```python
from build123d import *

# Parameters (mm, degrees)
SKETCH1_W            = 400
SKETCH1_H            = 800
BASE_DEPTH           = 18
SKETCH2_R            = 3.15
MOUNTING_HOLES_DEPTH = 19
TAP_HOLE_REACH       = 20
SKETCH4_R            = 8


with BuildPart() as part:
    # Sketch1 → Base (new body)
    with BuildSketch(Plane.XY):
        with Locations((200, 400)):
            Rectangle(SKETCH1_W, SKETCH1_H)
    extrude(amount=BASE_DEPTH)

    # Sketch2 → Mounting holes (cut, through all)
    with BuildSketch(Plane.XY.offset(18)):
        with Locations((25, 775)):
            Circle(SKETCH2_R)
        with Locations((375, 775)):
            Circle(SKETCH2_R)
        with Locations((25, 150)):
            Circle(SKETCH2_R)
        with Locations((375, 150)):
            Circle(SKETCH2_R)
    extrude(amount=-MOUNTING_HOLES_DEPTH, mode=Mode.SUBTRACT)

    # Sketch4 → Tap hole (cut, up to next)
    with BuildSketch(Plane(origin=(0, 0, 0), x_dir=(-1, 0, 0), z_dir=(0, 0, -1)), mode=Mode.PRIVATE) as tap_hole_sk1:
        with Locations((-75, 75)):
            Circle(SKETCH4_R)
    tap_hole_tool1 = extrude(tap_hole_sk1.sketch, amount=-TAP_HOLE_REACH, mode=Mode.PRIVATE) & part.part
    add(tap_hole_tool1.solids().sort_by_distance((75, 75, 0))[0], mode=Mode.SUBTRACT)


solid = part.part
```
Part model, mm, in its own coordinate system. Round coordinates to 2 decimals unless told otherwise and drop trailing zeros. Order: outer loops, then holes, each group sorted by start corner. A loop starts at its lowest first (then second) coordinate and runs counter-clockwise, first axis right, second up. Notation, with made-up numbers: M 31,-18.5 L 52,-18.5 A27 ccw 52,8.5 Z; hole C -13,41 d6. An arc over 180 degrees is marked long. Answer in a Markdown table with one row per item. Add a question column.
Q1. Cut at B-B on x = 75. Give the cut face in (y, z).
Q2. Cut at A-A on y = 75. Give the cut face in (x, z).
Q3. Pin check, flat tips, straight feed: pin 1 (5 mm diameter, centred on x = 25, y = 150, fed in from +Z); pin 2 (10 mm diameter, centred on x = 281, y = 330.5, fed in from -Z). Stop position of each tip, or through.
Q4. Wall check: L1, parallel to Y at x = 25, z = 6.25; L2, parallel to X at y = 150, z = 3.75; L3, parallel to Y at x = 69, z = 15.5. Give the ranges that are in metal, low to high. Write a range as from..to.
Q5. Mould opens along Y. For faces 1 (the face through (197, 800, 9)), 2 (the face through (197, 0, 9)), 3 (the face through (76.041, 82.932, 8.874)), 4 (the face through (197, 406, 18)) say: +Y half, -Y half, draft (parallel to the pull), parting line (faces both ways), or undercut.
Established:
| question | item | result |
|---|---|---|
| 1 | outline | M 0,0 L 67,0 L 67,18 L 0,18 Z; M 83,0 L 800,0 L 800,18 L 83,18 Z |
| 2 | outline | M 0,0 L 67,0 L 67,18 L 0,18 Z; M 83,0 L 400,0 L 400,18 L 83,18 Z |
| 3 | pin 1 | passes through |
| 3 | pin 2 | stops at z = 0 |
| 4 | L1 | y = 0..146.85, 153.15..771.85, 778.15..800 |
| 4 | L2 | x = 0..21.85, 28.15..371.85, 378.15..400 |
| 4 | L3 | y = 0..69.71, 80.29..800 |
| 5 | face 1 | +Y half |
| 5 | face 2 | -Y half |
| 5 | face 3 | undercut |
| 5 | face 4 | draft |
